Here's the drawing with two shaded views (mm, measured from the low corner). I have some questions. A direction names the side the tool comes from. Round coordinates to 2 decimals unless told otherwise and drop trailing zeros. Loops run counter-clockwise (first coordinate to the right, second up) from the corner with the lowest first, then second, coordinate; pieces in that order, holes last. Notation, with made-up numbers: (-30.5, -34.5) -> (0.5, -34.5) arc R26 ccw to (0.5, 3.5) -> close; hole circle Ø7 at (52.25, 6.25). An arc over 180 degrees is marked (long way). One line per item, written item: value. Start each with the question number.
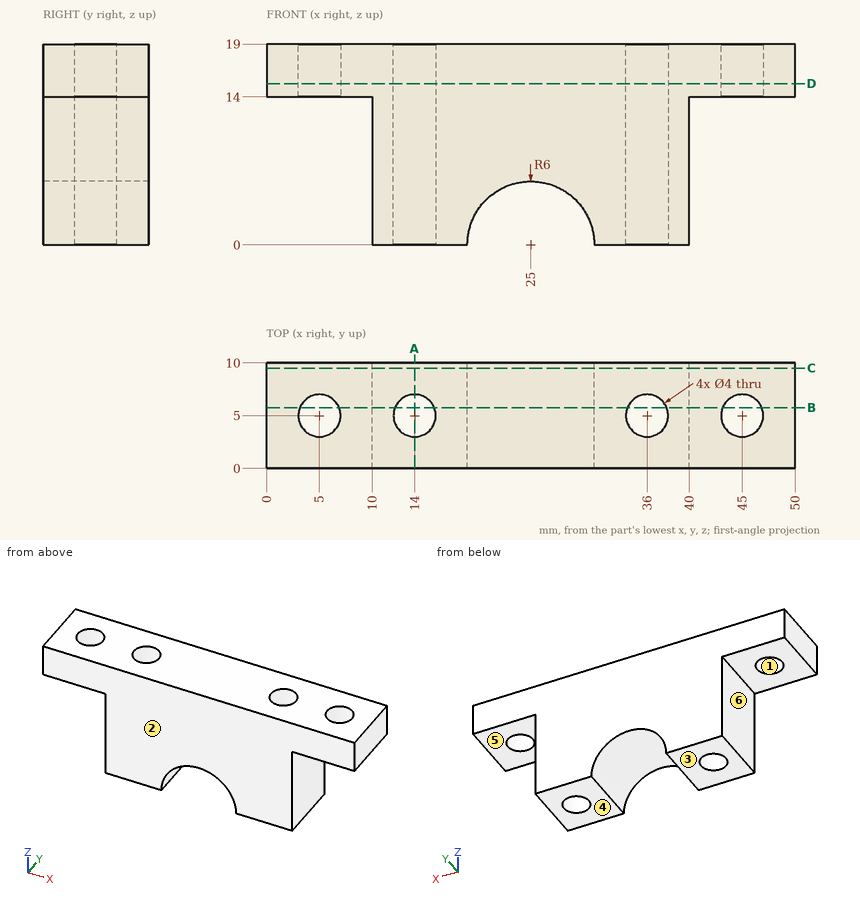
Q1. I want a section at D-D on z = 15.25. Please give me the cut outline in (x, y), plus the area to 3 significant figures.
Q2. Which directions (+Z, -Z, +X, -X, +Y, -Y) give clear straight access to the entire face, cutting with the end or side of a thin tool? Please do the marked faces 4, 5 and 6.
Q3. I want a section at B-B on y = 5.75. Please give me the cut outline in (x, z).
Q4. I want a section at C-C on y = 9.5. Please give me the cut outline in (x, z).
Q5. If I drill on line 1 along Y through (x, z) = (14, 9.25); line 2 along X through (y, z) = (4.5, 7.5); line 3 along X through (y, z) = (6.5, 10.25), over which ranges is the centre line in solid material (lowest first)?
Q6. I want a section at A-A on x = 14. Please give me the cut outline in (y, z), plus the area to 3 significant figures.
Q7. Will these pins go through, and if not, where does the flat tip stop? P1, Ø3.5, axis at x = 36, y = 5, coming from the -Z side; P2, Ø5, axis at x = 7, y = 6.5, coming from the -Z side; P3, Ø3, axis at x = 10, z = 12, coming from the -Y side; P4, Ø1, axis at y = 1.5, z = 3, coming from the +X side.
Q8. If we mould it in two halves opening along Y, with no side actions, what happens to the marked faces 1, 2 and 3? For each: released by +Y, released by -Y, zero draft, split by the parting line, or undercut.
Answers below:
1. outline: (0, 0) -> (50, 0) -> (50, 10) -> (0, 10) -> close; hole circle Ø4 at (5, 5); hole circle Ø4 at (14, 5); hole circle Ø4 at (36, 5); hole circle Ø4 at (45, 5)
1. area: 450 mm^2
2. face 4: -Z, +X, -X, +Y, -Y
2. face 5: -Z, +X, +Y, -Y
2. face 6: -Z, -X, +Y, -Y
3. outline: (0, 14) -> (3.15, 14) -> (3.15, 19) -> (0, 19) -> close; (6.85, 14) -> (10, 14) -> (10, 0) -> (12.15, 0) -> (12.15, 19) -> (6.85, 19) -> close; (15.85, 0) -> (19, 0) arc R6 cw to (31, 0) -> (34.15, 0) -> (34.15, 19) -> (15.85, 19) -> close; (37.85, 0) -> (40, 0) -> (40, 14) -> (43.15, 14) -> (43.15, 19) -> (37.85, 19) -> close; (46.85, 14) -> (50, 14) -> (50, 19) -> (46.85, 19) -> close
4. outline: (0, 14) -> (10, 14) -> (10, 0) -> (19, 0) arc R6 cw to (31, 0) -> (40, 0) -> (40, 14) -> (50, 14) -> (50, 19) -> (0, 19) -> close
5. line 1: y = 0 to 3, 7 to 10
5. line 2: x = 10 to 12.06, 15.94 to 34.06, 37.94 to 40
5. line 3: x = 10 to 12.68, 15.32 to 34.68, 37.32 to 40
6. outline: (0, 0) -> (3, 0) -> (3, 19) -> (0, 19) -> close; (7, 0) -> (10, 0) -> (10, 19) -> (7, 19) -> close
6. area: 114 mm^2
7. P1: passes through
7. P2: stops at z = 14
7. P3: stops at y = 0
7. P4: stops at x = 40
8. face 1: undercut
8. face 2: released by -Y
8. face 3: zero draft
